Design review of the part built by this model. Coordinates are the model's own, in mm. A direction names the side the tool comes from. Coordinates: 2 decimals unless noted, no trailing zeros. Loops run counter-clockwise (first coordinate to the right, second up) from the corner with the lowest first, then second, coordinate; pieces in that order, holes last.
Q1. Add section C-C on z = 19. Give the boundary of the cut face in (x, y).
Q2. Wall thickness on probe 1 along Y at (x, z) = (0, 44); probe 2 along X at (y, z) = (16, 39.5); probe 3 along Y at (x, z) = (6, 32.5): over which ranges is each line inside the solid? List them lowest first.
Q3. Add section D-D on y = 38. Give the boundary of the cut face in (x, z), and give its area (3 significant figures).
Q4. Add section A-A on y = 0. Give the boundary of the cut face in (x, z).
Q5. For P1, Ø6, axis at x = 46, y = 26, coming from the -Z side; P2, Ø3, axis at y = -14, z = 23, coming from the +X side; P3, Ø6, axis at x = 54.5, y = 0, coming from the +Z side, all flat-tipped, find the tip position at first contact; note any pin that passes through.
Q6. Draft analysis for pull direction Y (two halves, no side actions). For faces 1 (the face through (-1, -50, 49)), 2 (the face through (23.846, 7.509, 50.7)), 3 (the face through (50, -23, 58)), state which applies: released by +Y, released by -Y, zero draft, split by the parting line, or undercut.
Q7. Machinability: for faces 4 (the face through (-45, -1, 5)), 5 (the face through (62.325, -5.42, 22.417)), which of the approach directions +Z, -Z, +X, -X, +Y, -Y give a long, thin tool a straight path to every point of the face, cutting with its end or side? Answer none if there is none.
Q8. Add section B-B on x = 0. Give the boundary of the cut face in (y, z), and give its area (3 significant figures).
```python
from build123d import *

# Parameters (mm, degrees)
F0_W     = 100
F0_H     = 100
F1_DEPTH = 100
F2_R     = 10
F3_SIZE  = 10
F4_R     = 25
F5_DEPTH = 100
F6_R     = 25
F7_DEPTH = 25


with BuildPart() as f1:
    # F0 (on Top) → F1 (new body)
    with BuildSketch(Plane.XY):
        Rectangle(F0_W, F0_H)
    extrude(amount=F1_DEPTH)

    # F2
    f2_edges = [f1.edges().sort_by_distance(p)[0] for p in [
        (-50, 0, 100),
        (0, -50, 100),
        (50, 0, 100),
        (0, 50, 100),
    ]]
    fillet(f2_edges, radius=F2_R)

    # F3
    f3_edges = [f1.edges().sort_by_distance(p)[0] for p in [
        (0, -50, 0),
        (50, 0, 0),
        (0, 50, 0),
        (-50, 0, 0),
    ]]
    chamfer(f3_edges, length=F3_SIZE)

    # F4 (on face) → F5 (cut)
    with BuildSketch(Plane.XY.offset(100)):
        Circle(F4_R)
    extrude(amount=-F5_DEPTH, mode=Mode.SUBTRACT)

    # F6 (on face) → F7 (join)
    with BuildSketch(Plane.YZ.offset(50)):
        with Locations((0, 46.822905)):
            Circle(F6_R)
    extrude(amount=F7_DEPTH)


solid = f1.part
```
Entries:
1. outline: (-50, -50) - (50, -50) - (50, 50) - (-50, 50) - close; hole circle Ø50 at (0, 0)
2. probe 1: y = -50 to -25, 25 to 50
2. probe 2: x = -50 to -19.21, 19.21 to 75
2. probe 3: y = -50 to -24.27, 24.27 to 50
3. outline: (-50, 10) - (-40, 0) - (40, 0) - (50, 10) - (50, 90) arc R10 ccw to (40, 100) - (-40, 100) arc R10 ccw to (-50, 90) - close
3. area: 9,860 mm2
4. outline: (-50, 10) - (-40, 0) - (-25, 0) - (-25, 100) - (-40, 100) arc R10 ccw to (-50, 90) - close; (25, 0) - (40, 0) - (50, 10) - (50, 21.82) - (75, 21.82) - (75, 71.82) - (50, 71.82) - (50, 90) arc R10 ccw to (40, 100) - (25, 100) - close
5. P1: stops at z = 3
5. P2: stops at x = 50
5. P3: stops at z = 71.82
6. face 1: released by -Y
6. face 2: undercut
6. face 3: zero draft
7. face 4: -Z, -X, +Y, -Y
7. face 5: +X
8. outline: (-50, 10) - (-40, 0) - (-25, 0) - (-25, 100) - (-40, 100) arc R10 ccw to (-50, 90) - close; (25, 0) - (40, 0) - (50, 10) - (50, 90) arc R10 ccw to (40, 100) - (25, 100) - close
8. area: 4,860 mm2
